Part model, mm, in its own coordinate system. A direction names the side the tool comes from. Give positions to 0.01 mm unless a question says otherwise; leave off trailing zeros. Write each loop counter-clockwise with the first axis right and the second up, starting at its lowest first coordinate (ties: lowest second). Pieces come first, ordered by that corner, then holes.
from build123d import *

# Parameters (mm, degrees)
F0_R      = 8
F1_DEPTH  = 10.6
F2_W      = 19
F2_H      = 6.5
F3_DEPTH  = 10.6
F4_R      = 5.35
F5_DEPTH  = 10.601
F6_W      = 5.4454011573
F6_H      = 3
F7_DEPTH  = 10.601
F8_R      = 1.75
F9_DEPTH  = 16.001
F10_W     = 7
F10_H     = 10.6
F11_DEPTH = 26
F12_W     = 7
F12_H     = 10
F13_DEPTH = 25.5
F14_W     = 7
F14_H     = 10.6
F15_DEPTH = 26
F16_W     = 7
F16_H     = 10
F17_DEPTH = 25.5
F18_R     = 1.75
F19_DEPTH = 10


with BuildPart() as f1:
    # F0 (on Top) → F1 (new body)
    with BuildSketch(Plane.XY):
        Circle(F0_R)
    extrude(amount=-F1_DEPTH)

    # F2 (on face) → F3 (join, through all)
    with BuildSketch(Plane.XY):
        with Locations((-9.5, 4.75)):
            Rectangle(F2_W, F2_H)
        with Locations((-9.5, -4.75)):
            Rectangle(F2_W, F2_H)
    extrude(amount=-F3_DEPTH)

    # F4 (on face) → F5 (cut, through all)
    with BuildSketch(Plane.XY):
        Circle(F4_R)
    extrude(amount=-F5_DEPTH, mode=Mode.SUBTRACT)

    # F6 (on face) → F7 (cut, through all)
    with BuildSketch(Plane.XY):
        with Locations((-7.8581168228, 0)):
            Rectangle(F6_W, F6_H)
    extrude(amount=-F7_DEPTH, mode=Mode.SUBTRACT)

    # F8 (on face) → F9 (cut, through all)
    with BuildSketch(Plane.XZ.offset(8)):
        with Locations((-13.75, -5.25)):
            Circle(F8_R)
    extrude(amount=-F9_DEPTH, mode=Mode.SUBTRACT)

    # F10 (on face) → F11 (join)
    with BuildSketch(Plane.XZ.offset(8)):
        with Locations((-3.5, -5.3)):
            Rectangle(F10_W, F10_H)
    extrude(amount=F11_DEPTH)

    # F12 (on face) → F13 (join)
    with BuildSketch(Plane(origin=(0, 0, -10.6), x_dir=(1, 0, 0), z_dir=(0, 0, -1))):
        with Locations((-3.5, 29)):
            Rectangle(F12_W, F12_H)
    extrude(amount=F13_DEPTH)

    # F14 (on face) → F15 (join)
    with BuildSketch(Plane(origin=(0, 8, 0), x_dir=(-1, 0, 0), z_dir=(0, 1, 0))):
        with Locations((3.5, -5.3)):
            Rectangle(F14_W, F14_H)
    extrude(amount=F15_DEPTH)

    # F16 (on face) → F17 (join)
    with BuildSketch(Plane(origin=(0, 0, -10.6), x_dir=(1, 0, 0), z_dir=(0, 0, -1))):
        with Locations((-3.5, -29)):
            Rectangle(F16_W, F16_H)
    extrude(amount=F17_DEPTH)

    # F18 (on face) → F19 (cut)
    with BuildSketch(Plane(origin=(0, 0, -36.1), x_dir=(1, 0, 0), z_dir=(0, 0, -1))):
        with Locations((-3.5, 29)):
            Circle(F18_R)
        with Locations((-3.5, -29)):
            Circle(F18_R)
    extrude(amount=-F19_DEPTH, mode=Mode.SUBTRACT)


solid = f1.part
1) Saw through at D-D (z = -24). Write the cut outline in (x, y).
Check result:
outline: (-7, -34) - (0, -34) - (0, -24) - (-7, -24) - close; (-7, 24) - (0, 24) - (0, 34) - (-7, 34) - close
2) Flat gauge pins, fed straight in: P1, Ø13, axis at y = -18.5, z = -14.5, coming from the +X side; P2, Ø2, axis at x = -3.5, y = -29, coming from the -Z side; P3, Ø8, axis at x = -9, z = -15, coming from the -Y side; P4, Ø12, axis at x = -12.5, y = 10.5, coming from the -Z side. Where does each tip first touch, or does it go through?
Check result:
P1: stops at x = 0
P2: stops at z = -26.1
P3: stops at y = -34
P4: stops at z = -10.6
3) Saw through at B-B (x = -9.75). Write the cut outline in (y, z), and give its area (3 significant figures).
Check result:
outline: (-8, -10.6) - (-1.5, -10.6) - (-1.5, 0) - (-8, 0) - close; (1.5, -10.6) - (8, -10.6) - (8, 0) - (1.5, 0) - close
area: 138 mm2
4) Mould opens along Y. For faces 1 (the flat face through (0, 27, -14)), 2 (the flat face through (-11.8, -8, -5.2)), 3 (the flat face through (-4, 24, -23)) say: +Y half, -Y half, draft (parallel to the pull), parting line (faces both ways), or undercut.
Check result:
face 1: draft
face 2: -Y half
face 3: undercut
5) Saw through at C-C (y = -29). Write the cut outline in (x, z), and give its area (3 significant figures).
Check result:
outline: (-7, -36.1) - (-5.25, -36.1) - (-5.25, -26.1) - (-1.75, -26.1) - (-1.75, -36.1) - (0, -36.1) - (0, 0) - (-7, 0) - close
area: 218 mm2
6) 3-axis set-ups, long thin cutter, end or side, ignore diameter. For faces 4 (the flat face through (-12, -1.5, -4)), 5 (the flat face through (-11.8, 8, -5.2)), 6 (the cylindrical face through (-5.25, -29.08, -31.17)): which of +Z, -Z, +X, -X, +Y, -Y reach the whole face in a straight line?
Check result:
face 4: +Z, -Z, -X
face 5: +Z, -Z, -X, +Y
face 6: -Z
7) Saw through at A-A (z = -5.25). Write the cut outline in (x, y).
Check result:
outline: (-19, -8) - (-15.5, -8) - (-15.5, -1.5) - (-19, -1.5) - close; (-19, 1.5) - (-15.5, 1.5) - (-15.5, 8) - (-19, 8) - close; (-12, -8) - (-7, -8) - (-7, -34) - (0, -34) - (0, -8) arc R8 ccw to (0, 8) - (0, 34) - (-7, 34) - (-7, 8) - (-12, 8) - (-12, 1.5) - (-5.14, 1.5) arc R5.35 cw (long way) to (-5.14, -1.5) - (-12, -1.5) - close
8) Drill centre lines: L1, parallel to Y at x = -3.5, z = -31.5; L2, parallel to Y at x = -12.75, z = -2.5; L3, parallel to Y at x = -4.5, z = -24. Where is each one in solid material? Low to high.
Check result:
L1: y = -34 to -30.75, -27.25 to -24, 24 to 27.25, 30.75 to 34
L2: y = -8 to -1.5, 1.5 to 8
L3: y = -34 to -24, 24 to 34
